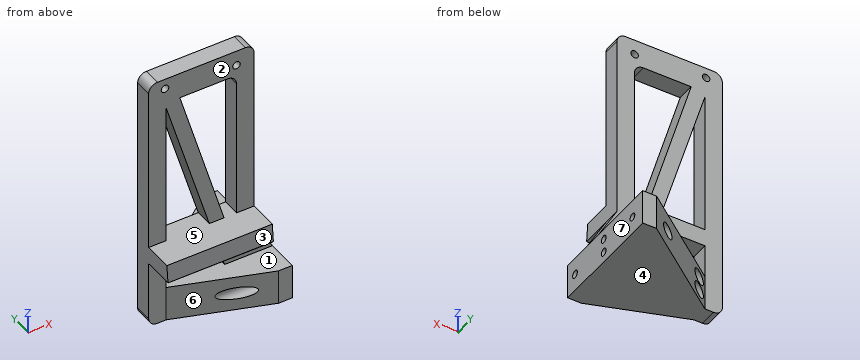
```python
from build123d import *

# Parameters (mm, degrees)
EXTRUDE_1_DEPTH                 = 10
SKETCH_4_W                      = 7.875
SKETCH_4_H                      = 20
EXTRUDE_2_DEPTH                 = 40
CUT_EXTRUDE_1_REACH             = 116.35
SKETCH_5_R                      = 2.15
CUT_EXTRUDE_1_DIRECTION_2_DEPTH = 53
CUT_EXTRUDE_2_REACH             = 107.272
SKETCH_6_R                      = 2.15
FILLET_1_R                      = 5
FILLET_2_R                      = 5
SKETCH_7_W                      = 7.875
SKETCH_7_H                      = 20
EXTRUDE_3_DEPTH                 = 18
CUT_EXTRUDE_3_REACH             = 116.35
SKETCH_8_R                      = 2.15
EXTRUDE_8_DEPTH                 = 20
SKETCH_15_W                     = 52.625
SKETCH_15_H                     = 20
EXTRUDE_9_DEPTH                 = 40
CUT_EXTRUDE_START               = -7.875
SKETCH_14_R                     = 3.5
CUT_EXTRUDE_8_DEPTH             = 54
CUT_EXTRUDE_10_DEPTH            = 20
EXTRUDE_10_DEPTH                = 10
EXTRUDE_11_DEPTH                = 17.5
CUT_EXTRUDE_11_DEPTH            = 64


with BuildPart() as part:
    # 草图1 → 凸台-拉伸1 (new body)
    with BuildSketch(Plane(origin=(0, 0, 0), x_dir=(1, 0, 0), z_dir=(0, 1, 0))):
        Polygon((5.931150433, 81.572237736), (53.180774799, 81.572237736), (53.180774799, 61.572237736), (42.680774799, 42.721022935), (42.680774799, 31.757290204), (42.680774799, -57.600660719), (42.680774799, -67.427762264), (0.431150433, -67.427762264), (-17.319225201, -67.427762264), (-17.319225201, 81.572237736), align=None)
        Polygon((47.930774799, 61.572237736), (42.680774799, 61.572237736), (42.680774799, 52.689495612), align=None, mode=Mode.SUBTRACT)
        Polygon((25.906315323, 61.572237736), (-7.319225201, 61.572237736), (-7.319225201, -49.220735683), align=None, mode=Mode.SUBTRACT)
        Polygon((0.431150433, -52.427762264), (32.680774799, -52.427762264), (32.680774799, 56.508121895), align=None, mode=Mode.SUBTRACT)
    extrude(amount=EXTRUDE_1_DEPTH)

    # 草图4 → 凸台-拉伸2 (add)
    with BuildSketch(Plane(origin=(0, 10, 0), x_dir=(1, 0, 0), z_dir=(0, 1, 0))):
        with Locations((49.243274799, 71.572237736)):
            Rectangle(SKETCH_4_W, SKETCH_4_H)
    extrude(amount=EXTRUDE_2_DEPTH)

    # 草图5 → 切除-拉伸1 (cut, up to next)
    with BuildSketch(Plane.ZY.offset(-45.305774799), mode=Mode.PRIVATE) as cut_extrude_1_sk1:
        with Locations(Location((-75.572237736, 14.7, 0), (0, 0, 180))):
            Circle(SKETCH_5_R)
    cut_extrude_1_tool1 = extrude(cut_extrude_1_sk1.sketch, amount=-CUT_EXTRUDE_1_REACH, mode=Mode.PRIVATE) & part.part
    # 草图5 → 切除-拉伸1 (cut, up to next)
    with BuildSketch(Plane.ZY.offset(-45.305774799), mode=Mode.PRIVATE) as cut_extrude_1_sk2:
        with Locations(Location((-67.572237736, 14.7, 0), (0, 0, 180))):
            Circle(SKETCH_5_R)
    cut_extrude_1_tool2 = extrude(cut_extrude_1_sk2.sketch, amount=-CUT_EXTRUDE_1_REACH, mode=Mode.PRIVATE) & part.part
    # 草图5 → 切除-拉伸1 (cut, up to next)
    with BuildSketch(Plane.ZY.offset(-45.305774799), mode=Mode.PRIVATE) as cut_extrude_1_sk3:
        with Locations(Location((-71.572237736, 40.7, 0), (0, 0, 180))):
            Circle(SKETCH_5_R)
    cut_extrude_1_tool3 = extrude(cut_extrude_1_sk3.sketch, amount=-CUT_EXTRUDE_1_REACH, mode=Mode.PRIVATE) & part.part
    add(cut_extrude_1_tool1.solids().sort_by_distance((45.305775, 14.7, -75.572238))[0], mode=Mode.SUBTRACT)
    add(cut_extrude_1_tool2.solids().sort_by_distance((45.305775, 14.7, -67.572238))[0], mode=Mode.SUBTRACT)
    add(cut_extrude_1_tool3.solids().sort_by_distance((45.305775, 40.7, -71.572238))[0], mode=Mode.SUBTRACT)

    # 草图5 → 切除-拉伸1 direction 2 (cut)
    with BuildSketch(Plane.ZY.offset(-45.305774799)):
        with Locations(Location((-75.572237736, 14.7, 0), (0, 0, 180))):
            Circle(SKETCH_5_R)
        with Locations(Location((-67.572237736, 14.7, 0), (0, 0, 180))):
            Circle(SKETCH_5_R)
        with Locations(Location((-71.572237736, 40.7, 0), (0, 0, 180))):
            Circle(SKETCH_5_R)
    extrude(amount=CUT_EXTRUDE_1_DIRECTION_2_DEPTH, mode=Mode.SUBTRACT)

    # 草图6 → 切除-拉伸2 (cut, up to next)
    with BuildSketch(Plane(origin=(0, 10, 0), x_dir=(1, 0, 0), z_dir=(0, 1, 0)), mode=Mode.PRIVATE) as cut_extrude_2_sk1:
        with Locations(Location((-8.019225201, -61.542634482, 0), (0, 0, 270))):
            Circle(SKETCH_6_R)
    cut_extrude_2_tool1 = extrude(cut_extrude_2_sk1.sketch, amount=-CUT_EXTRUDE_2_REACH, mode=Mode.PRIVATE) & part.part
    # 草图6 → 切除-拉伸2 (cut, up to next)
    with BuildSketch(Plane(origin=(0, 10, 0), x_dir=(1, 0, 0), z_dir=(0, 1, 0)), mode=Mode.PRIVATE) as cut_extrude_2_sk2:
        with Locations(Location((32.680774799, -58.692634482, 0), (0, 0, 270))):
            Circle(SKETCH_6_R)
    cut_extrude_2_tool2 = extrude(cut_extrude_2_sk2.sketch, amount=-CUT_EXTRUDE_2_REACH, mode=Mode.PRIVATE) & part.part
    add(cut_extrude_2_tool1.solids().sort_by_distance((-8.019225, 10, 61.542634))[0], mode=Mode.SUBTRACT)
    add(cut_extrude_2_tool2.solids().sort_by_distance((32.680775, 10, 58.692634))[0], mode=Mode.SUBTRACT)

    # 圆角1
    fillet_1_edges = [part.edges().sort_by_distance(p)[0] for p in [
        (-17.319225201, 5, 67.427762264),
        (-17.319225201, 5, -81.572237736),
        (42.680774799, 5, 67.427762264),
    ]]
    fillet(fillet_1_edges, radius=FILLET_1_R)

    # 圆角2
    fillet_2_edges = [part.edges().sort_by_distance(p)[0] for p in [
        (32.680774799, 5, 52.427762264),
    ]]
    fillet(fillet_2_edges, radius=FILLET_2_R)

    # 草图7 → 凸台-拉伸3 (add)
    with BuildSketch(Plane.XZ):
        with Locations((49.243274799, -71.572237736)):
            Rectangle(SKETCH_7_W, SKETCH_7_H)
    extrude(amount=EXTRUDE_3_DEPTH)

    # 草图8 → 切除-拉伸3 (cut, up to next)
    with BuildSketch(Plane.ZY.offset(-45.305774799), mode=Mode.PRIVATE) as cut_extrude_3_sk1:
        with Locations((-71.572237736, -11.3)):
            Circle(SKETCH_8_R)
    cut_extrude_3_tool1 = extrude(cut_extrude_3_sk1.sketch, amount=-CUT_EXTRUDE_3_REACH, mode=Mode.PRIVATE) & part.part
    add(cut_extrude_3_tool1.solids().sort_by_distance((45.305775, -11.3, -71.572238))[0], mode=Mode.SUBTRACT)

    # 草图13 → 凸台-拉伸8 (add)
    with BuildSketch(Plane.XY.offset(-61.572237736)):
        Polygon((45.305774799, 0), (45.305774799, -18), (-7.319225201, 0), align=None)
    extrude(amount=-EXTRUDE_8_DEPTH)

    # 草图15 → 凸台-拉伸9 (add)
    with BuildSketch(Plane(origin=(0, 10, 0), x_dir=(1, 0, 0), z_dir=(0, 1, 0))):
        with Locations((18.993274799, 71.572237736)):
            Rectangle(SKETCH_15_W, SKETCH_15_H)
    extrude(amount=EXTRUDE_9_DEPTH)

    # 草图14 → 切除-拉伸8 (cut)
    with BuildSketch(Plane(origin=(53.180774799, 0, 0), x_dir=(0, 0, -1), z_dir=(1, 0, 0)).offset(CUT_EXTRUDE_START)):
        with Locations((71.572237736, 40.7)):
            Circle(SKETCH_14_R)
        with Locations((67.572237736, 14.7)):
            Circle(SKETCH_14_R)
        with Locations((75.572237736, 14.7)):
            Circle(SKETCH_14_R)
        with Locations((71.572237736, -11.3)):
            Circle(SKETCH_14_R)
    extrude(amount=-CUT_EXTRUDE_8_DEPTH, mode=Mode.SUBTRACT)

    # 草图17 → 切除-拉伸10 (cut)
    with BuildSketch(Plane.XY.offset(-61.572237736)):
        Polygon((-7.319225201, 10), (-7.319225201, 50), (45.305774799, 50), align=None)
    extrude(amount=-CUT_EXTRUDE_10_DEPTH, mode=Mode.SUBTRACT)

    # 草图18 → 凸台-拉伸10 (add)
    with BuildSketch(Plane(origin=(0, 10, 0), x_dir=(1, 0, 0), z_dir=(0, 1, 0))):
        Polygon((-7.319225201, 32.572237736), (17.209548321, 32.572237736), (20.208433494, 42.572237736), (-7.319225201, 42.572237736), align=None)
        Polygon((25.594741772, 32.572237736), (32.680774799, 32.572237736), (32.680774799, 56.508121895), align=None)
        Polygon((42.680774799, 61.572237736), (42.680774799, 52.689495612), (47.930774799, 61.572237736), align=None)
    extrude(amount=-EXTRUDE_10_DEPTH)

    # 草图19 → 凸台-拉伸11 (add)
    with BuildSketch(Plane.XZ):
        Polygon((-17.319225201, -32.572237736), (-17.319225201, -42.572237736), (42.680774799, -42.721022935), (42.680774799, -32.572237736), align=None)
    extrude(amount=EXTRUDE_11_DEPTH)

    # 草图20 → 切除-拉伸11 (cut)
    with BuildSketch(Plane.ZY.offset(17.319225201)):
        Polygon((-42.572237736, -17.5), (-32.572237736, -17.5), (-32.572237736, -16.5), align=None)
    extrude(amount=-CUT_EXTRUDE_11_DEPTH, mode=Mode.SUBTRACT)


solid = part.part
```
Verification items for the finished model (mm, model axes). Face numbers are marked on the shaded views. A direction names the side the tool comes from. Round coordinates to 2 decimals unless told otherwise and drop trailing zeros. Order: outer loops, then holes, each group sorted by start corner. A loop starts at its lowest first (then second) coordinate and runs counter-clockwise, first axis right, second up. Notation, with made-up numbers: (-25, 59) -> (28, 59) arc R29 ccw to (28, 93) -> close; hole circle Ø7 at (70, 37). An arc over 180 degrees is marked (long way). Put each result on its own line as item: value. Start each with the question number.
(1) Section check B-B (z = -30). Enter the section's corners in (x, y).
(2) Depth check by flat-ended pin: pin 1 Ø4 at (x, z) = (-8.02, 61.54) entering from +Y; pin 2 Ø12 at (x, z) = (44, 48) entering from +Y; pin 3 Ø10 at (x, z) = (18.5, -28.5) entering from -Y; pin 4 Ø8 at (y, z) = (3, -56) entering from +X. Enter the tip coordinate at first touch or a pass-through.
(3) Section check C-C (y = 40.7). Enter the section's corners in (x, z).
(4) Draft check along Z on the marked faces 1, 2, 3 and 4. Enter one of: +Z half, -Z half, draft (parallel to the pull), parting line (faces both ways), or undercut.
(5) Tool access check on the marked faces 5, 6 and 7. Record the directions out of +Z, -Z, +X, -X, +Y, -Y that give a thin tool (end or side, any length) a straight path to the whole face; none if there is none.
(6) Material ranges on line 1 along Z through (x, y) = (28, 14.7); line 2 along Z through (x, y) = (32.75, -11.3); line 3 along Z through (x, y) = (8.5, -5), recorded low to high.
(7) Section check A-A (x = 14). Enter the section's corners in (y, z), then the cut area to 3 significant figures.
(8) Section check D-D (z = -55.5). Enter the section's corners in (x, y).
Completed:
1. outline: (-17.32, 0) -> (-7.32, 0) -> (-7.32, 10) -> (-17.32, 10) -> close; (16.44, 0) -> (24.83, 0) -> (24.83, 10) -> (16.44, 10) -> close; (32.68, 0) -> (42.68, 0) -> (42.68, 10) -> (32.68, 10) -> close
2. pin 1: passes through
2. pin 2: stops at y = 10
2. pin 3: stops at y = -16.59
2. pin 4: stops at x = 52.31
3. outline: (33.07, -81.57) -> (53.18, -81.57) -> (53.18, -73.72) -> (45.31, -73.72) -> (45.31, -75.07) -> (33.07, -75.07) -> close; (33.07, -68.07) -> (45.31, -68.07) -> (45.31, -69.42) -> (53.18, -69.42) -> (53.18, -61.57) -> (33.07, -61.57) -> close
4. face 1: undercut
4. face 2: draft
4. face 3: +Z half
4. face 4: -Z half
5. face 5: -Y
5. face 6: -Z, -X, -Y
5. face 7: +Z, -Z, +X, +Y, -Y
6. line 1: z = -81.57 to -79.07, -72.07 to -71.07, -64.07 to -61.57
6. line 2: z = -81.57 to -75.07, -68.07 to -61.57, -42.7 to -32.57
6. line 3: z = -81.57 to -61.57, -42.64 to -32.57
7. outline: (-17.5, -42.65) -> (0, -42.65) -> (0, -42.57) -> (10, -42.57) -> (10, -32.57) -> (-16.5, -32.57) -> (-17.5, -42.57) -> close; (-7.29, -81.57) -> (26.2, -81.57) -> (26.2, -61.57) -> (-7.29, -61.57) -> close; (0, -21.87) -> (10, -21.87) -> (10, 6.59) -> (0, 6.59) -> close; (0, 52.43) -> (10, 52.43) -> (10, 67.43) -> (0, 67.43) -> close; hole circle Ø7 at (14.7, -75.57); hole circle Ø7 at (14.7, -67.57)
7. area: 1,300 mm2
8. outline: (-17.32, 0) -> (-7.32, 0) -> (-7.32, 10) -> (-17.32, 10) -> close; (24.09, 0) -> (49.8, 0) -> (49.8, 10) -> (24.09, 10) -> close
